Autodesk Inventor part; units mm, degrees
ref_plane "YZ Plane" through (0, 0, 0) normal (1, 0, 0) x (0, 1, 0)
ref_plane "XZ Plane" through (0, 0, 0) normal (0, 1, 0) x (-1, 0, 0)
ref_plane "XY Plane" through (0, 0, 0) normal (0, 0, 1) x (1, 0, 0)
sketch "Schizzo1" plane through (0, 0, 0) normal (0, 1, 0) x (-1, 0, 0)
  line L0 (-14.5, 5) -> (-14.5, 9.5)
  line L1 (-14.5, 9.5) -> (-11, 9.5)
  line L2 (-11, 9.5) -> (-11, 8.5)
  line L3 (-11, 8.5) -> (-9.7, 8.5)
  line L4 (-9.7, 8.5) -> (-9.7, 9.5)
  line L5 (-9.7, 9.5) -> (0, 9.5)
  line L6 (0, 9.5) -> (0, 5)
  line L7 (0, 5) -> (-14.5, 5)
  line L8 (0, 0) -> (5.7518, 0)
  dimension "d0" = 10
  dimension "d2" = 19
  dimension "d3" = 14.5
  dimension "d4" = 11
  dimension "d5" = 1.3
  dimension "d6" = 17
revolve "Rivoluzione1" add sketch "Schizzo1" angle 360 about axis through (0, 0, 0) along (-1, 0, 0)
fillet "Raccordo1" radius 1 1 edges at (14.5, 0, -9.5)
sketch "Schizzo2" plane through (14.5, 0, 0) normal (1, 0, 0) x (0, 0, -1)
  circle A0 centre (0, 0) radius 8.5
  circle A1 centre (0, 0) radius 7.1007
extrude "Estrusione2" cut sketch "Schizzo2" against normal blind 1 contours A1
mirror "Specchio1" about plane through (0, 0, 7.25) normal (-1, 0, 0)
properties part number "LM10UU"
Source: CAD feature listing. Evaluate the final solid. Frame: model axes, mm. A direction names the side the tool comes from. Round coordinates to 2 decimals unless told otherwise and drop trailing zeros. Write each loop counter-clockwise with the first axis right and the second up, starting at its lowest first coordinate (ties: lowest second). Pieces come first, ordered by that corner, then holes. Notation, with made-up numbers: M 85.5,-27.75 L 118.5,-27.75 A20 cw 118.5,-14.75 Z; hole C 43,88 d8. An arc over 180 degrees is marked long. One line per item, written item: value. Start each with the question number.
Item 1: Mould query, pull axis Z, two halves, no side actions, for faces 1 (the cylindrical face through (0.19, 4.88, -1.08)), 2 (the cylindrical face through (-12.23, 8.43, 4.38)), 3 (the flat face through (9.7, -8.4, -2.2)). Classes: pulls with the +Z half, pulls with the -Z half, needs draft (parallel to the pull), parting line crosses it, or undercut.
Item 2: Section query B-B (x = -10.5). Return the cut outline in (y, z), plus the area to 3 significant figures.
Item 3: Ray query, L1, parallel to X at y = 8.5, z = -1; L2, parallel to Y at x = 4.5, z = 0; L3, parallel to X at y = 2.5, z = 4.5. Return the intervals inside material, ascending. Write a range as from..to.
Item 4: Set-up query: faces 4 (the cylindrical face through (10.341, 7.167, 4.57)), 5 (the cylindrical face through (14.01, -6.93, 1.54)), 6 (the flat face through (-13.5, 5, -2)). Return all of +Z, -Z, +X, -X, +Y, -Y with unobstructed straight access to the full face (end or side cutting, diameter ignored); none if empty.
Item 5: Pin query (flat end, axial travel): pin 1 (4 mm diameter, centred on x = 6, z = -7.5, fed in from -Y); pin 2 (5 mm diameter, centred on y = -5, z = 2.5, fed in from +X); pin 3 (7 mm diameter, centred on y = 1, z = 2, fed in from -X); pin 4 (10 mm diameter, centred on x = 1.5, y = -5.5, fed in from -Z). Return the tip coordinate at first contact, or that it passes through.
Item 6: Section query A-A (x = 1.75). Return the cut outline in (y, z), plus the area to 3 significant figures.
Result set:
1. face 1: undercut
1. face 2: parting line crosses it
1. face 3: needs draft
2. outline: C 0,0 d17; hole C 0,0 d10
2. area: 148 mm²
3. L1: x = -14.5..-11, -9.7..9.7, 11..14.5
3. L2: y = -9.5..-5, 5..9.5
3. L3: x = -13.5..13.5
4. face 4: none
4. face 5: +X
4. face 6: -X
5. pin 1: stops at y = -7.75
5. pin 2: stops at x = 14.5
5. pin 3: stops at x = -13.5
5. pin 4: stops at z = -9.49
6. outline: C 0,0 d19; hole C 0,0 d10
6. area: 205 mm²
